```python
from build123d import *

# Parameters (mm, degrees)
SKETCH_2_R          = 35
SKETCH_2_R_2        = 5.5
EXTRUDE_1_DEPTH     = 5
EXTRUDE_START       = 15
SKETCH_3_R          = 35
SKETCH_3_R_2        = 30.1
EXTRUDE_2_DEPTH     = 15
SKETCH_4_R          = 1.55
CUT_EXTRUDE_1_DEPTH = 10
CUT_EXTRUDE_5_DEPTH = 15
FILLET_1_R          = 1
CUT_EXTRUDE_START   = -2
SKETCH_10_R         = 35
CUT_EXTRUDE_6_DEPTH = 2
CUT_EXTRUDE_7_DEPTH = 10
SKETCH5_R           = 1.55
CUT_EXTRUDE2_DEPTH  = 2


with BuildPart() as part:
    # 草图2 → 凸台-拉伸1 (new body)
    with BuildSketch(Plane.XY):
        Circle(SKETCH_2_R)
        Circle(SKETCH_2_R_2, mode=Mode.SUBTRACT)
    extrude(amount=EXTRUDE_1_DEPTH)

    # 草图3 → 凸台-拉伸2 (add)
    with BuildSketch(Plane(origin=(0, 0, 0), x_dir=(-1, 0, 0), z_dir=(0, 0, -1)).offset(EXTRUDE_START)):
        Circle(SKETCH_3_R)
        Circle(SKETCH_3_R_2, mode=Mode.SUBTRACT)
    extrude(amount=-EXTRUDE_2_DEPTH)

    # 草图4 → 切除-拉伸1 (cut)
    with BuildSketch(Plane(origin=(0, 0, -15), x_dir=(-1, 0, 0), z_dir=(0, 0, -1))):
        with Locations((0, 32.5)):
            Circle(SKETCH_4_R)
        with Locations((32.5, 0)):
            Circle(SKETCH_4_R)
        with Locations((0, -32.5)):
            Circle(SKETCH_4_R)
        with Locations((-32.5, 0)):
            Circle(SKETCH_4_R)
    extrude(amount=-CUT_EXTRUDE_1_DEPTH, mode=Mode.SUBTRACT)

    # 草图9 → 切除-拉伸5 (cut)
    with BuildSketch(Plane(origin=(0, 0, -15), x_dir=(-1, 0, 0), z_dir=(0, 0, -1))):
        with BuildLine():
            ThreePointArc((-22.013313369, 20.528615017), (-22.026376234, 22.026376234), (-20.528615017, 22.013313369))
            ThreePointArc((-20.528615017, 22.013313369), (-21.283914114, 21.283914114), (-22.013313369, 20.528615017))
        make_face()
        with BuildLine():
            ThreePointArc((20.528615017, 22.013313369), (22.026376234, 22.026376234), (22.013313369, 20.528615017))
            ThreePointArc((22.013313369, 20.528615017), (21.283914114, 21.283914114), (20.528615017, 22.013313369))
        make_face()
        with BuildLine():
            ThreePointArc((22.013313369, -20.528615017), (22.026376234, -22.026376234), (20.528615017, -22.013313369))
            ThreePointArc((20.528615017, -22.013313369), (21.283914114, -21.283914114), (22.013313369, -20.528615017))
        make_face()
        with BuildLine():
            ThreePointArc((-20.528615017, -22.013313369), (-22.026376234, -22.026376234), (-22.013313369, -20.528615017))
            ThreePointArc((-22.013313369, -20.528615017), (-21.283914114, -21.283914114), (-20.528615017, -22.013313369))
        make_face()
    extrude(amount=-CUT_EXTRUDE_5_DEPTH, mode=Mode.SUBTRACT)

    # 圆角1
    # the kernel refuses this fillet: 1 mm, written as the material it takes off along each edge
    with BuildSketch(Plane(origin=(0, 0, -15), x_dir=(-0.7403558797037455, 0.6722151228498904, 0), z_dir=(-0.6722151228498904, -0.7403558797037455, 0))) as fillet_1_piece_1:
        with BuildLine():
            CenterArc((30.1 + FILLET_1_R, -FILLET_1_R), FILLET_1_R, 90, 90)
            Line((30.1, -FILLET_1_R), (30.1, 0))
            Line((30.1, 0), (30.1 + FILLET_1_R, 0))
        make_face()
    revolve(axis=Axis((0, 0, -15), (0, 0, -1)), revolution_arc=95.523479776, mode=Mode.SUBTRACT)
    with BuildSketch(Plane(origin=(0, 0, -15), x_dir=(0.6722151228498918, 0.7403558797037441, 0), z_dir=(-0.7403558797037441, 0.6722151228498918, 0))) as fillet_1_piece_2:
        with BuildLine():
            CenterArc((30.1 + FILLET_1_R, -FILLET_1_R), FILLET_1_R, 90, 90)
            Line((30.1, -FILLET_1_R), (30.1, 0))
            Line((30.1, 0), (30.1 + FILLET_1_R, 0))
        make_face()
    revolve(axis=Axis((0, 0, -15), (0, 0, -1)), revolution_arc=95.523479776, mode=Mode.SUBTRACT)
    with BuildSketch(Plane(origin=(0, 0, -15), x_dir=(0.7403558797037453, -0.6722151228498905, 0), z_dir=(0.6722151228498905, 0.7403558797037453, 0))) as fillet_1_piece_3:
        with BuildLine():
            CenterArc((30.1 + FILLET_1_R, -FILLET_1_R), FILLET_1_R, 90, 90)
            Line((30.1, -FILLET_1_R), (30.1, 0))
            Line((30.1, 0), (30.1 + FILLET_1_R, 0))
        make_face()
    revolve(axis=Axis((0, 0, -15), (0, 0, -1)), revolution_arc=95.523479776, mode=Mode.SUBTRACT)
    with BuildSketch(Plane(origin=(0, 0, -15), x_dir=(-1, 0, 0), z_dir=(0, -1, 0))) as fillet_1_piece_4:
        with BuildLine():
            CenterArc((30.1 + FILLET_1_R, -FILLET_1_R), FILLET_1_R, 90, 90)
            Line((30.1, -FILLET_1_R), (30.1, 0))
            Line((30.1, 0), (30.1 + FILLET_1_R, 0))
        make_face()
    revolve(axis=Axis((0, 0, -15), (0, 0, -1)), revolution_arc=47.760430641, mode=Mode.SUBTRACT)
    with BuildSketch(Plane(origin=(0, 0, -15), x_dir=(-0.6722320403041436, -0.7403405189428228, 0), z_dir=(0.7403405189428228, -0.6722320403041436, 0))) as fillet_1_piece_5:
        with BuildLine():
            CenterArc((30.1 + FILLET_1_R, -FILLET_1_R), FILLET_1_R, 90, 90)
            Line((30.1, -FILLET_1_R), (30.1, 0))
            Line((30.1, 0), (30.1 + FILLET_1_R, 0))
        make_face()
    revolve(axis=Axis((0, 0, -15), (0, 0, -1)), revolution_arc=47.760430641, mode=Mode.SUBTRACT)

    # 草图10 → 切除-拉伸6 (cut)
    with BuildSketch(Plane.XY.offset(5).offset(CUT_EXTRUDE_START)):
        with Locations(Location((0, 0, 0), (0, 0, 180))):
            Circle(SKETCH_10_R)
    extrude(amount=CUT_EXTRUDE_6_DEPTH, mode=Mode.SUBTRACT)

    # 草图11 → 切除-拉伸7 (cut)
    with BuildSketch(Plane(origin=(0, 0, 0), x_dir=(-1, 0, 0), z_dir=(0, 0, -1))):
        with BuildLine():
            Line((12.990381057, 7.5), (15.588457268, 9))
            ThreePointArc((15.588457268, 9), (18, 0), (15.588457268, -9))
            Line((15.588457268, -9), (12.990381057, -7.5))
            ThreePointArc((12.990381057, -7.5), (15, 0), (12.990381057, 7.5))
        make_face()
        with BuildLine():
            Line((-7.5, 12.990381057), (-9, 15.588457268))
            ThreePointArc((-9, 15.588457268), (0, 18), (9, 15.588457268))
            Line((9, 15.588457268), (7.5, 12.990381057))
            ThreePointArc((7.5, 12.990381057), (0, 15), (-7.5, 12.990381057))
        make_face()
        with BuildLine():
            Line((7.5, -12.990381057), (9, -15.588457268))
            ThreePointArc((9, -15.588457268), (0, -18), (-9, -15.588457268))
            Line((-9, -15.588457268), (-7.5, -12.990381057))
            ThreePointArc((-7.5, -12.990381057), (0, -15), (7.5, -12.990381057))
        make_face()
        with BuildLine():
            Line((-12.990381057, -7.5), (-15.588457268, -9))
            ThreePointArc((-15.588457268, -9), (-18, 0), (-15.588457268, 9))
            Line((-15.588457268, 9), (-12.990381057, 7.5))
            ThreePointArc((-12.990381057, 7.5), (-15, 0), (-12.990381057, -7.5))
        make_face()
    extrude(amount=-CUT_EXTRUDE_7_DEPTH, mode=Mode.SUBTRACT)

    # Sketch5 → Cut-Extrude2 (cut)
    with BuildSketch(Plane.XY.offset(3)):
        with Locations((8.838834765, 8.838834765)):
            Circle(SKETCH5_R)
        with Locations((8.838834765, -8.838834765)):
            Circle(SKETCH5_R)
        with Locations((-8.838834765, -8.838834765)):
            Circle(SKETCH5_R)
        with Locations((-8.838834765, 8.838834765)):
            Circle(SKETCH5_R)
    extrude(amount=-CUT_EXTRUDE2_DEPTH, mode=Mode.SUBTRACT)


solid = part.part
```
The listing builds one solid part. Answer for the finished solid, in the listing's coordinates (mm). A direction names the side the tool comes from. Round coordinates to 2 decimals unless told otherwise and drop trailing zeros. Write each loop counter-clockwise with the first axis right and the second up, starting at its lowest first coordinate (ties: lowest second). Pieces come first, ordered by that corner, then holes. Notation, with made-up numbers: (2, 43.25) -> (18, 43.25) arc R18 cw to (18, 72.25) -> close; hole circle Ø8 at (40.25, 62.5). An arc over 180 degrees is marked (long way). Answer as a JSON object with one key per item and string values. Group by question number.
Q1. Section A-A (z = -9) is taken. Write down the section's boundary in (x, y).
Q2. Which of the six approach directions +Z, -Z, +X, -X, +Y, -Y give full straight-line access (tool end or side, diameter ignored) to faces 1 (the face through (-8.26, 14.31, 1.48)), 2 (the face through (9, 9, 1)), 3 (the face through (-0.3, 30.1, -7.1))?
Q3. Section B-B (y = 32.5) is taken. Write down the section's boundary in (x, z), plus the area to 3 significant figures.
Q4. Determine the mould class of faces 4 (the face through (2.8, 31.3, -15)), 5 (the face through (30.1, 0.3, -7.1)) for opening direction Y: pulls with the +Y half, pulls with the -Y half, needs draft (parallel to the pull), parting line crosses it, or undercut.
Q5. Each of these flat-tipped pins is pushed along its axis until it touches: pin 1 Ø5 at (x, y) = (-8.84, 8.84) entering from +Z; pin 2 Ø3 at (x, y) = (8.84, 8.84) entering from -Z; pin 3 Ø3 at (y, z) = (-9, -4) entering from -X; pin 4 Ø1 at (y, z) = (-4.5, -3.5) entering from -X. Where does it stop, or does it pass through?
Q6. Section D-D (y = 4) is taken. Count the separate pieces of the cut face and the enclosed holes in it, plus the area to 3 significant figures.
Q7. Straight lines are drawn through the part: line 1 along Y through (x, z) = (0, -8.75); line 2 along X through (y, z) = (0, 0.9); line 3 along X through (y, z) = (32.5, -10.5). For each, find the intervals that lie inside material, in ascending order.
Check values:
{
 "1": {"outline": "circle Ø70 at (0, 0); hole circle Ø3.1 at (-32.5, 0); hole (-22.01, -20.53) arc R1.05 ccw (long way) to (-20.53, -22.01) arc R30.1 ccw to (20.53, -22.01) arc R1.05 ccw (long way) to (22.01, -20.53) arc R30.1 ccw to (22.01, 20.53) arc R1.05 ccw (long way) to (20.53, 22.01) arc R30.1 ccw to (-20.53, 22.01) arc R1.05 ccw (long way) to (-22.01, 20.53) arc R30.1 ccw to start; hole circle Ø3.1 at (0, -32.5); hole circle Ø3.1 at (0, 32.5); hole circle Ø3.1 at (32.5, 0)"},
 "2": {"face 1": "+Z, -Z", "face 2": "+Z", "face 3": "-Z"},
 "3": {"outline": "(-12.99, -15) -> (-1.55, -15) -> (-1.55, -5) -> (1.55, -5) -> (1.55, -15) -> (12.99, -15) -> (12.99, 3) -> (-12.99, 3) -> close", "area": "437 mm^2"},
 "4": {"face 4": "needs draft", "face 5": "undercut"},
 "5": {"pin 1": "z = 3", "pin 2": "z = 0", "pin 3": "x = -34.19", "pin 4": "x = -34.77"},
 "6": {"separate pieces": "4", "enclosed holes": "0", "area": "315 mm^2"},
 "7": {"line 1": "-35 to -34.05, -30.95 to -30.1, 30.1 to 30.95, 34.05 to 35", "line 2": "-35 to -18, -15 to -5.5, 5.5 to 15, 18 to 35", "line 3": "-12.99 to -1.55, 1.55 to 12.99"}
}
